from build123d import *

# Parameters (mm, degrees)
F0_W     = 76.2
F0_H     = 50.8
F1_DEPTH = 25.4
F2_SIZE  = 5.08
F3_R     = 5.08


with BuildPart() as f1:
    # F0 (on Top) → F1 (new body)
    with BuildSketch(Plane.XY):
        with Locations((38.1, -25.4)):
            Rectangle(F0_W, F0_H)
    extrude(amount=F1_DEPTH)

    # F2
    f2_edges = [f1.edges().sort_by_distance(p)[0] for p in [
        (38.1, -50.8, 25.4),
        (0, -25.4, 25.4),
        (38.1, 0, 25.4),
    ]]
    chamfer(f2_edges, length=F2_SIZE)

    # F3
    f3_edges = [f1.edges().sort_by_distance(p)[0] for p in [
        (40.64, -5.08, 25.4),
        (5.08, -25.4, 25.4),
        (40.64, -45.72, 25.4),
    ]]
    fillet(f3_edges, radius=F3_R)


solid = f1.part
Work out the finished part from the listing and answer in its coordinate system (mm). Give positions to 0.01 mm unless a question says otherwise; leave off trailing zeros. Loops run counter-clockwise (first coordinate to the right, second up) from the corner with the lowest first, then second, coordinate; pieces in that order, holes last. Notation, with made-up numbers: (48, 63.5) -> (78, 63.5) arc R3 cw to (78, 68.5) -> close; hole circle Ø9 at (59, -13.5). An arc over 180 degrees is marked (long way). Use a Markdown table: item, result. Add a question column.
1. Section A-A on x = 67 is taken. Determine the outline of the cut face in (y, z), and give its area (3 significant figures).
2. Find the intervals of material crossed by probe 1 along X at (y, z) = (-16.5, 22.25); probe 2 along X at (y, z) = (-23.5, 23.5); probe 3 along Z at (x, y) = (22, -47.5), in increasing order.
3. Section B-B on z = 22.5 is taken. Determine the outline of the cut face in (x, y), and give its area (3 significant figures).
Results below:
| question | item | result |
|---|---|---|
| 1 | outline | (-50.8, 0) -> (0, 0) -> (0, 20.32) -> (-3.59, 23.91) arc R5.08 ccw to (-7.18, 25.4) -> (-43.62, 25.4) arc R5.08 ccw to (-47.21, 23.91) -> (-50.8, 20.32) -> close |
| 1 | area | 1,260 mm^2 |
| 2 | probe 1 | x = 1.93 to 76.2 |
| 2 | probe 2 | x = 3.18 to 76.2 |
| 2 | probe 3 | z = 0 to 23.62 |
| 3 | outline | (2.18, -48.62) -> (76.2, -48.62) -> (76.2, -2.18) -> (2.18, -2.18) -> close |
| 3 | area | 3,440 mm^2 |
